Read the model definition and answer for the solid it produces. Units are mm, in the model's axes. Face numbers are marked on the shaded views. Give positions to 0.01 mm unless a question says otherwise; leave off trailing zeros. Loops run counter-clockwise (first coordinate to the right, second up) from the corner with the lowest first, then second, coordinate; pieces in that order, holes last.
(1) Find section C-C, the plane y = -1.25. Write down the section's boundary in (x, z), then the cut area to 3 significant figures.
(2) Find section D-D, the plane x = 20.5. Write down the section's boundary in (y, z).
(3) Find section B-B, the plane z = 2.65. Write down the section's boundary in (x, y), then the cut area to 3 significant figures.
(4) Find section A-A, the plane x = -21.5. Write down the section's boundary in (y, z).
(5) Straight lines are drawn through the part: probe 1 along Y at (x, z) = (21.5, 2.45); probe 2 along Y at (x, z) = (-21.5, 2.05); probe 3 along X at (y, z) = (1.5, 1.1). For each, find the intervals that lie inside material, in ascending order.
(6) Each of these flat-tipped pins is pushed along its axis until it touches: P1, Ø2, axis at x = -11, y = 4, coming from the -Z side; P2, Ø1.5, axis at y = 5, z = 3.5, coming from the +X side. Where does it stop, or does it pass through?
(7) Determine the mould class of the marked faces 1, 2, 3 and 4 for opening direction X: pulls with the +X half, pulls with the -X half, needs draft (parallel to the pull), parting line crosses it, or undercut.
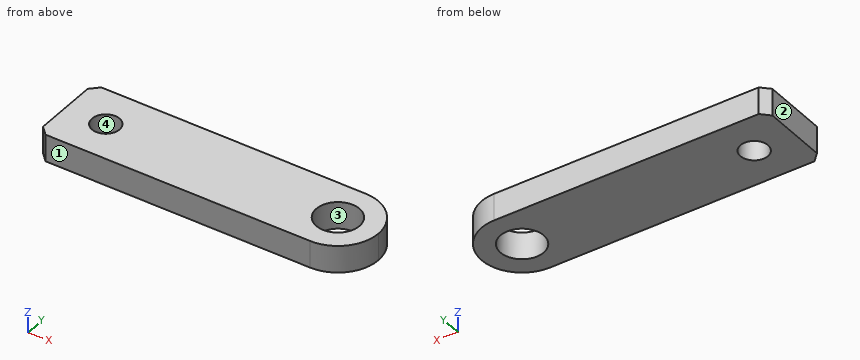
```python
from build123d import *

# Parameters (mm, degrees)
F0_R     = 2.55
F0_R_2   = 4
F1_DEPTH = 5
F2_SIZE  = 1.5


with BuildPart() as f1:
    # F0 (on Top) → F1 (new body)
    with BuildSketch(Plane.XY):
        with BuildLine():
            Line((-29, -7.5), (21.5, -7.5))
            ThreePointArc((21.5, -7.5), (26.803301, -5.303301), (29, 0))
            ThreePointArc((29, 0), (26.803301, 5.303301), (21.5, 7.5))
            Line((21.5, 7.5), (-29, 7.5))
            Line((-29, 7.5), (-29, -7.5))
        make_face()
        with Locations((-21.5, 0)):
            Circle(F0_R, mode=Mode.SUBTRACT)
        with Locations((21.5, 0)):
            Circle(F0_R_2, mode=Mode.SUBTRACT)
    extrude(amount=F1_DEPTH)

    # F2
    f2_edges = [f1.edges().sort_by_distance(p)[0] for p in [
        (-29, 7.5, 2.5),
        (-29, -7.5, 2.5),
    ]]
    chamfer(f2_edges, length=F2_SIZE)


solid = f1.part
```
Entries:
1. outline: (-29, 0) - (-23.72, 0) - (-23.72, 5) - (-29, 5) - close; (-19.28, 0) - (17.7, 0) - (17.7, 5) - (-19.28, 5) - close; (25.3, 0) - (28.9, 0) - (28.9, 5) - (25.3, 5) - close
1. area: 229 mm2
2. outline: (-7.5, 0) - (-3.87, 0) - (-3.87, 5) - (-7.5, 5) - close; (3.87, 0) - (7.5, 0) - (7.5, 5) - (3.87, 5) - close
3. outline: (-29, -6) - (-27.5, -7.5) - (21.5, -7.5) arc R7.5 ccw to (21.5, 7.5) - (-27.5, 7.5) - (-29, 6) - close; hole circle Ø5.1 at (-21.5, 0); hole circle Ø8 at (21.5, 0)
3. area: 773 mm2
4. outline: (-7.5, 0) - (-2.55, 0) - (-2.55, 5) - (-7.5, 5) - close; (2.55, 0) - (7.5, 0) - (7.5, 5) - (2.55, 5) - close
5. probe 1: y = -7.5 to -4, 4 to 7.5
5. probe 2: y = -7.5 to -2.55, 2.55 to 7.5
5. probe 3: x = -29 to -23.56, -19.44 to 17.79, 25.21 to 28.85
6. P1: stops at z = 0
6. P2: stops at x = 27.68
7. face 1: needs draft
7. face 2: pulls with the -X half
7. face 3: undercut
7. face 4: undercut
